```python
from build123d import *

# Parameters (mm, degrees)
SKETCH1_R           = 1.5
BOSS_EXTRUDE1_DEPTH = 10
BOSS_EXTRUDE2_DEPTH = 3
SKETCH3_R           = 1.5
BOSS_EXTRUDE3_DEPTH = 6


with BuildPart() as part:
    # Sketch1 → Boss-Extrude1 (new body)
    with BuildSketch(Plane(origin=(0, 0, 0), x_dir=(1, 0, 0), z_dir=(0, 1, 0))):
        Polygon((2.598076211, 0), (1.299038106, 2.25), (-1.299038106, 2.25), (-2.598076211, 0), (-1.299038106, -2.25), (1.299038106, -2.25), align=None)
        with Locations(Location((0, 0, 0), (0, 0, 270))):
            Circle(SKETCH1_R, mode=Mode.SUBTRACT)
    extrude(amount=BOSS_EXTRUDE1_DEPTH)

    # Sketch2 → Boss-Extrude2 (add)
    with BuildSketch(Plane(origin=(0, 10, 0), x_dir=(1, 0, 0), z_dir=(0, 1, 0))):
        Polygon((2.598076211, 0), (1.299038106, 2.25), (-1.299038106, 2.25), (-2.598076211, 0), (-1.299038106, -2.25), (1.299038106, -2.25), align=None)
    extrude(amount=-BOSS_EXTRUDE2_DEPTH)

    # Sketch3 → Boss-Extrude3 (add)
    with BuildSketch(Plane(origin=(0, 10, 0), x_dir=(1, 0, 0), z_dir=(0, 1, 0))):
        with Locations(Location((0, 0, 0), (0, 0, 270))):
            Circle(SKETCH3_R)
    extrude(amount=BOSS_EXTRUDE3_DEPTH)


solid = part.part
```
Model file for the job. Use its own axes, mm. A direction names the side the tool comes from. Coordinates: 2 decimals unless noted, no trailing zeros. Order: outer loops, then holes, each group sorted by start corner. A loop starts at its lowest first (then second) coordinate and runs counter-clockwise, first axis right, second up. Notation, with made-up numbers: (42.5, 41.5) -> (99.5, 41.5) arc R26 ccw to (99.5, 68.5) -> close; hole circle Ø5 at (35.25, 72). An arc over 180 degrees is marked (long way). Answer as a JSON object with one key per item and string values. Group by question number.
1) Pull direction Z, two halves, no side cores. Call faces 1 (the face through (0, 7, 0)), 2 (the face through (0, 5, 2.25)), 3 (the face through (0, 16, 0)): +Z half, -Z half, draft (parallel to the pull), parting line (faces both ways), or undercut.
2) Drill centre lines: L1, parallel to Z at x = 0, y = 3; L2, parallel to Y at x = 1, z = -0.9; L3, parallel to X at y = 5.25, z = -1.15. Where is each one in solid material? Low to high.
3) Cut at C-C, the plane z = 0.25. Write the cut outline in (x, y), then the cut area to 3 significant figures.
4) Cut at B-B, the plane x = 0. Write the cut outline in (y, z).
5) Flat gauge pin, fed straight in: pin 1 (2 mm diameter, centred on x = -1, y = 14, fed in from -Z). Where does the tip first touch, or does it go through?
6) Which spindle directions (+Z, -Z, +X, -X, +Y, -Y) get a long thin tool onto all of the face, cutting with end or side? Do faces 4 (the face through (0.45, 3.45, 1.43)), 5 (the face through (0, 5, -2.25)), 6 (the face through (0.45, 12.96, 1.43)). Say none if no direction does.
7) Cut at A-A, the plane y = 5.5. Write the cut outline in (x, z).
8) Cut at D-D, the plane y = 9.75. Write the cut outline in (x, z).
Check values:
{
 "1": {"face 1": "undercut", "face 2": "+Z half", "face 3": "draft"},
 "2": {"L1": "z = -2.25 to -1.5, 1.5 to 2.25", "L2": "y = 7 to 16", "L3": "x = -1.93 to -0.96, 0.96 to 1.93"},
 "3": {"outline": "(-2.45, 0) -> (-1.48, 0) -> (-1.48, 7) -> (1.48, 7) -> (1.48, 0) -> (2.45, 0) -> (2.45, 10) -> (1.48, 10) -> (1.48, 16) -> (-1.48, 16) -> (-1.48, 10) -> (-2.45, 10) -> close", "area": "46.1 mm²"},
 "4": {"outline": "(0, -2.25) -> (10, -2.25) -> (10, -1.5) -> (16, -1.5) -> (16, 1.5) -> (10, 1.5) -> (10, 2.25) -> (0, 2.25) -> (0, 1.5) -> (7, 1.5) -> (7, -1.5) -> (0, -1.5) -> close"},
 "5": {"pin 1": "stops at z = -1.5"},
 "6": {"face 4": "-Y", "face 5": "-Z, +X, -X, +Y, -Y", "face 6": "+Y"},
 "7": {"outline": "(-2.6, 0) -> (-1.3, -2.25) -> (1.3, -2.25) -> (2.6, 0) -> (1.3, 2.25) -> (-1.3, 2.25) -> close; hole circle Ø3 at (0, 0)"},
 "8": {"outline": "(-2.6, 0) -> (-1.3, -2.25) -> (1.3, -2.25) -> (2.6, 0) -> (1.3, 2.25) -> (-1.3, 2.25) -> close"}
}
